Verification items for the finished model (mm, model axes). A direction names the side the tool comes from. Give positions to 0.01 mm unless a question says otherwise; leave off trailing zeros. Order: outer loops, then holes, each group sorted by start corner. A loop starts at its lowest first (then second) coordinate and runs counter-clockwise, first axis right, second up.
from build123d import *

# Parameters (mm, degrees)
F0_W     = 80
F0_H     = 75
F0_R     = 3.25
F1_DEPTH = 12
F2_R     = 5.5
F3_DEPTH = 6
F4_R     = 2.5
F5_DEPTH = 20
F6_R     = 2.5
F7_DEPTH = 20
F8_R     = 2.5
F9_DEPTH = 20


with BuildPart() as f1:
    # F0 (on Front) → F1 (new body)
    with BuildSketch(Plane.XZ):
        with Locations((40, 37.5)):
            Rectangle(F0_W, F0_H)
        with Locations((15, 25)):
            Circle(F0_R, mode=Mode.SUBTRACT)
        with Locations((65, 25)):
            Circle(F0_R, mode=Mode.SUBTRACT)
    extrude(amount=F1_DEPTH)

    # F2 (on face) → F3 (cut)
    with BuildSketch(Plane(origin=(0, 0, 0), x_dir=(-1, 0, 0), z_dir=(0, 1, 0))):
        with Locations((-15, 25)):
            Circle(F2_R)
        with Locations((-65, 25)):
            Circle(F2_R)
    extrude(amount=-F3_DEPTH, mode=Mode.SUBTRACT)

    # F4 (on face) → F5 (cut)
    with BuildSketch(Plane(origin=(0, 0, 0), x_dir=(1, 0, 0), z_dir=(0, 0, -1))):
        with Locations((15, 6)):
            Circle(F4_R)
        with Locations((65, 6)):
            Circle(F4_R)
    extrude(amount=-F5_DEPTH, mode=Mode.SUBTRACT)

    # F6 (on face) → F7 (cut)
    with BuildSketch(Plane.XY.offset(75)):
        with Locations((15, -6)):
            Circle(F6_R)
        with Locations((65, -6)):
            Circle(F6_R)
    extrude(amount=-F7_DEPTH, mode=Mode.SUBTRACT)

    # F8 (on face) → F9 (cut)
    with BuildSketch(Plane(origin=(0, 0, 0), x_dir=(0, -1, 0), z_dir=(-1, 0, 0))):
        with Locations((6, 62.5)):
            Circle(F8_R)
        with Locations((6, 12.5)):
            Circle(F8_R)
    extrude(amount=-F9_DEPTH, mode=Mode.SUBTRACT)


solid = f1.part
(1) Section check D-D, the plane y = -7. Give the number of separate pieces and of enclosed holes in the cut face, then the cut area to 3 significant figures.
Solved:
separate pieces: 3
enclosed holes: 2
area: 5,430 mm2
(2) Go/stop test with flat-tipped pins: pin 1 (1 mm diameter, centred on x = 15.5, y = -7.5, fed in from -Z); pin 2 (3 mm diameter, centred on x = 65, y = -6, fed in from +Z); pin 3 (5 mm diameter, centred on x = 65.5, z = 27.5, fed in from +Y). Record where each tip stops, or that it passes through.
Solved:
pin 1: stops at z = 20
pin 2: stops at z = 55
pin 3: stops at y = -6
(3) Section check B-B, the plane y = -1.5. Enter the section's corners in (x, z).
Solved:
outline: (0, 0) - (80, 0) - (80, 75) - (0, 75) - close; hole circle Ø11 at (15, 25); hole circle Ø11 at (65, 25)
(4) Section check A-A, the plane x = 65. Enter the section's corners in (y, z), then the cut area to 3 significant figures.
Solved:
outline: (-12, 0) - (-8.5, 0) - (-8.5, 20) - (-6, 20) - (-6, 21.75) - (-12, 21.75) - close; (-12, 28.25) - (-6, 28.25) - (-6, 30.5) - (0, 30.5) - (0, 75) - (-3.5, 75) - (-3.5, 55) - (-8.5, 55) - (-8.5, 75) - (-12, 75) - close; (-3.5, 0) - (0, 0) - (0, 19.5) - (-3.5, 19.5) - close
area: 596 mm2
(5) Scan lines: line 1 (X direction, y = -9.7, z = 25); line 2 (Z direction, x = 9, y = -6); line 3 (X direction, y = -6, z = 5). Record each from-to range of solid material in increasing order.
Solved:
line 1: x = 0 to 11.75, 18.25 to 61.75, 68.25 to 80
line 2: z = 0 to 10, 15 to 60, 65 to 75
line 3: x = 0 to 12.5, 17.5 to 62.5, 67.5 to 80
(6) Section check C-C, the plane z = 17.5. Enter the section's corners in (x, y), then the cut area to 3 significant figures.
Solved:
outline: (0, -12) - (80, -12) - (80, 0) - (0, 0) - close; hole circle Ø5 at (15, -6); hole circle Ø5 at (65, -6)
area: 921 mm2
(7) Set-up check for faces 4 (the cylindrical face through (12.5, -5.9, 58)), 5 (the cylindrical face through (67.385, -6.751, 9.86)), 6 (the cylindrical face through (65.716, -2.958, 30.453)), 7 (the cylindrical face through (7, -6, 15)), 8 (the flat face through (39, -6, 0)): record each of +Z, -Z, +X, -X, +Y, -Y from which the full face is reachable in a straight line by a thin tool's end or side.
Solved:
face 4: +Z
face 5: -Z
face 6: +Y
face 7: -X
face 8: -Z, +X, -X, +Y, -Y
(8) Release check for a two-part mould opening along Y. For faces 1 (the flat face through (39, -6, 75)), 2 (the cylindrical face through (12.5, -6.1, 4.8)), 3 (the flat face through (39, 0, 38)) record: pulls with the +Y half, pulls with the -Y half, needs draft (parallel to the pull), parting line crosses it, or undercut.
Solved:
face 1: needs draft
face 2: undercut
face 3: pulls with the +Y half
